Here's how the part is built. I have some questions about the finished solid (model axes, mm). Face numbers are marked on the shaded views. A direction names the side the tool comes from. Coordinates: 2 decimals unless noted, no trailing zeros. Write each loop counter-clockwise with the first axis right and the second up, starting at its lowest first coordinate (ties: lowest second). Pieces come first, ordered by that corner, then holes. Notation, with made-up numbers: M 84.25,69.5 L 139.25,69.5 A17 ccw 139.25,90.5 Z; hole C 69.25,66.25 d6. An arc over 180 degrees is marked long. Use one line per item in the form item = value. Start each with the question number.
1. I want a section at A-A, the plane y = -15.5. List the corners of the cut face in (x, z) for me, plus the area to 3 significant figures.
2. I want a section at C-C, the plane y = 15.5. List the corners of the cut face in (x, z) for me.
3. Please list where these lines run through material, in increasing order: line 1 along Y through (x, z) = (-15.5, 3); line 2 along Z through (x, y) = (7, 6). Write a range as [from, to].
4. On a 3-axis mill with a long thin cutter (end or side, diameter ignored), from which of +Z, -Z, +X, -X, +Y, -Y can I reach the whole of each face in a straight line? I mean the marked faces 1, 2, 3, 4 and 5. Say none if no direction works.
5. I'm going to push flat-ended pins straight in: pin 1 Ø2.5 at (x, y) = (14.5, 16) entering from -Z; pin 2 Ø2 at (x, z) = (-7.5, 7) entering from +Y. Where does each tip first touch, or does it pass through?
6. Thinking about a two-plate mould opening in X: for the marked faces 6, 7, 8 and 9, which applies, released by +X, released by -X, zero draft, split by the parting line, or undercut?
7. I want a section at D-D, the plane z = 10.25. List the corners of the cut face in (x, y) for me.
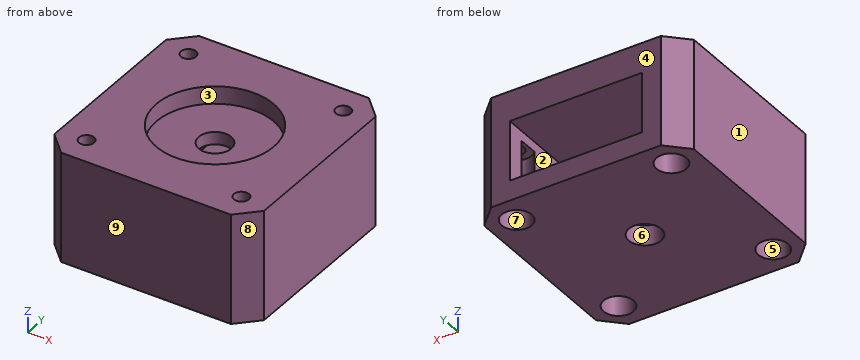
from build123d import *

# Parameters (mm, degrees)
F0_W      = 42
F0_H      = 42
F1_DEPTH  = 22
F2_SIZE   = 4
F3_R      = 11.75
F4_DEPTH  = 3.5
F5_R      = 3.25
F6_DEPTH  = 18.501
F8_START  = -4
F8_DEPTH  = 12
F9_R      = 1.5
F10_DEPTH = 22.001
F11_R     = 3
F12_DEPTH = 14


with BuildPart() as f1:
    # F0 (on Top) → F1 (new body)
    with BuildSketch(Plane.XY):
        Rectangle(F0_W, F0_H)
    extrude(amount=F1_DEPTH)

    # F2
    f2_edges = [f1.edges().sort_by_distance(p)[0] for p in [
        (-21, -21, 11),
        (21, -21, 11),
        (-21, 21, 11),
        (21, 21, 11),
    ]]
    chamfer(f2_edges, length=F2_SIZE)

    # F3 (on face) → F4 (cut)
    with BuildSketch(Plane.XY.offset(22)):
        Circle(F3_R)
    extrude(amount=-F4_DEPTH, mode=Mode.SUBTRACT)

    # F5 (on face) → F6 (cut, through all)
    with BuildSketch(Plane.XY.offset(18.5)):
        Circle(F5_R)
    extrude(amount=-F6_DEPTH, mode=Mode.SUBTRACT)

    # F7 (on face) → F8 (cut)
    with BuildSketch(Plane(origin=(0, 0, 0), x_dir=(1, 0, 0), z_dir=(0, 0, -1)).offset(F8_START)):
        with BuildLine():
            Line((-13.25, 0), (-13.25, -21))
            Line((-13.25, -21), (13.25, -21))
            Line((13.25, -21), (13.25, 0))
            ThreePointArc((13.25, 0), (0, 13.25), (-13.25, 0))
        make_face()
    extrude(amount=-F8_DEPTH, mode=Mode.SUBTRACT)

    # F9 (on face) → F10 (cut, through all)
    with BuildSketch(Plane.XY.offset(22)):
        with Locations((-15.5, 15.5)):
            Circle(F9_R)
        with Locations((15.5, 15.5)):
            Circle(F9_R)
        with Locations((-15.5, -15.5)):
            Circle(F9_R)
        with Locations((15.5, -15.5)):
            Circle(F9_R)
    extrude(amount=-F10_DEPTH, mode=Mode.SUBTRACT)

    # F11 (on face) → F12 (cut)
    with BuildSketch(Plane(origin=(0, 0, 0), x_dir=(1, 0, 0), z_dir=(0, 0, -1))):
        with Locations((-15.5, 15.5)):
            Circle(F11_R)
        with Locations((15.5, 15.5)):
            Circle(F11_R)
        with Locations((-15.5, -15.5)):
            Circle(F11_R)
        with Locations((15.5, -15.5)):
            Circle(F11_R)
    extrude(amount=-F12_DEPTH, mode=Mode.SUBTRACT)


solid = f1.part
Answer list:
q1.outline = M -21,0 L -18.5,0 L -18.5,14 L -17,14 L -17,22 L -21,22 Z; M -14,14 L -12.5,14 L -12.5,0 L 12.5,0 L 12.5,14 L 14,14 L 14,22 L -14,22 Z; M 17,14 L 18.5,14 L 18.5,0 L 21,0 L 21,22 L 17,22 Z
q1.area = 708 mm²
q2.outline = M -21,0 L -18.5,0 L -18.5,14 L -17,14 L -17,22 L -21,22 Z; M -14,14 L -13.25,14 L -13.25,16 L 13.25,16 L 13.25,14 L 14,14 L 14,22 L -14,22 Z; M -12.5,0 L 12.5,0 L 12.5,4 L -12.5,4 Z; M 17,14 L 18.5,14 L 18.5,0 L 21,0 L 21,22 L 17,22 Z
q3.line_1 = [-21, -18.5], [-12.5, 12.5], [18.5, 21]
q3.line_2 = [0, 4], [16, 18.5]
q4.face_1 = +Z, -Z, -X, +Y, -Y
q4.face_2 = +Y
q4.face_3 = +Z
q4.face_4 = +Z, -Z, +X, -X, +Y
q4.face_5 = -Z
q5.pin_1 = 14
q5.pin_2 = -10.16
q6.face_6 = undercut
q6.face_7 = undercut
q6.face_8 = released by +X
q6.face_9 = zero draft
q7.outline = M -21,-17 L -17,-21 L 17,-21 L 21,-17 L 21,17 L 17,21 L 13.25,21 L 13.25,17.48 A3 cw long 13.25,13.52 L 13.25,0 A13.25 cw -13.25,0 L -13.25,13.52 A3 cw long -13.25,17.48 L -13.25,21 L -17,21 L -21,17 Z; hole C -15.5,-15.5 d6; hole C 15.5,-15.5 d6
